from build123d import *

# Parameters (mm, degrees)
SKETCH2_W           = 24
SKETCH2_H           = 24
BOSS_EXTRUDE2_DEPTH = 50
SKETCH4_R           = 1.4
CUT_EXTRUDE1_DEPTH  = 8
CHAMFER1_SIZE       = 2
CHAMFER2_SIZE       = 4


with BuildPart() as part:
    # Sketch2 → Boss-Extrude2 (new body)
    with BuildSketch(Plane.XY):
        with Locations((12, 12)):
            Rectangle(SKETCH2_W, SKETCH2_H)
    extrude(amount=BOSS_EXTRUDE2_DEPTH)

    # Sketch4 → Cut-Extrude1 (cut)
    with BuildSketch(Plane(origin=(0, 0, 0), x_dir=(-1, 0, 0), z_dir=(0, 0, -1))):
        with Locations((-21, 21)):
            Circle(SKETCH4_R)
        with Locations((-21, 3)):
            Circle(SKETCH4_R)
        with Locations((-3, 3)):
            Circle(SKETCH4_R)
        with Locations((-3, 21)):
            Circle(SKETCH4_R)
    extrude(amount=-CUT_EXTRUDE1_DEPTH, mode=Mode.SUBTRACT)

    # Chamfer1
    chamfer1_edges = [part.edges().sort_by_distance(p)[0] for p in [
        (0, 24, 25),
        (24, 24, 25),
        (24, 0, 25),
        (0, 0, 25),
    ]]
    chamfer(chamfer1_edges, length=CHAMFER1_SIZE)

    # Chamfer2
    # the kernel refuses this chamfer: 4 mm, written as the material it takes off along each edge
    with BuildSketch(Plane(origin=(-8.286731952, 0, 50), x_dir=(0, -0.02749587661058639, -0.9996219169112968), z_dir=(1, 0, 0))) as chamfer2_piece_1:
        Polygon((CHAMFER2_SIZE * 0.999621916911, CHAMFER2_SIZE * 0.0274958766106), (-CHAMFER2_SIZE * 0.0274958766106, CHAMFER2_SIZE * 0.999621916911), (0, 0), align=None)
    extrude(amount=40.573463904, mode=Mode.SUBTRACT)
    with BuildSketch(Plane(origin=(24, -8.286731952, 50), x_dir=(-0.9996219169112968, 0, 0.027495876610585623), z_dir=(0, 1, 0)), Plane(origin=(32.286731952, 24, 50), x_dir=(0, -0.9996219169112968, 0.027495876610585623), z_dir=(-1, 0, 0)), Plane(origin=(0, 32.286731952, 50), x_dir=(0.9996219169112968, 0, 0.02749587661058563), z_dir=(0, -1, 0))) as chamfer2_piece_2:
        Polygon((CHAMFER2_SIZE * 0.999621916911, -CHAMFER2_SIZE * 0.0274958766106), (-CHAMFER2_SIZE * 0.0274958766106, -CHAMFER2_SIZE * 0.999621916911), (0, 0), align=None)
    extrude(amount=40.573463904, mode=Mode.SUBTRACT)


solid = part.part
Geometry: final body of the model. Coordinates: model frame, mm. A direction names the side the tool comes from. Give positions to 0.01 mm unless a question says otherwise; leave off trailing zeros. Loops run counter-clockwise (first coordinate to the right, second up) from the corner with the lowest first, then second, coordinate; pieces in that order, holes last. Notation, with made-up numbers: M 16.25,59 L 22.25,59 A24 ccw 22.25,80 Z; hole C -21,39.5 d7. An arc over 180 degrees is marked long. Put each result on its own line as item: value. Start each with the question number.
1) Pull-direction query (Y, two-part tool) for faces 1 (the flat face through (23, 1, 23)), 2 (the cylindrical face through (20.35, 19.76, 3.94)), 3 (the flat face through (12, 24, 23)), 4 (the cylindrical face through (3.303, 19.633, 3.944)); classes: pulls with the +Y half, pulls with the -Y half, needs draft (parallel to the pull), parting line crosses it, or undercut.
2) Cut plane A-A (z = 3.5). Output: boundary loops of the cut face in (x, y).
3) Ray query, line 1 along Y through (x, z) = (21, 4.75); line 2 along Y through (x, z) = (11, 48); line 3 along Z through (x, y) = (22, 16.5). Return the intervals inside material, ascending.
4) Cut plane B-B (y = 21). Output: boundary loops of the cut face in (x, z).
5) Access query for faces 5 (the flat face through (3, 3, 8)), 6 (the flat face through (12, 12, 0)). Directions: +Z, -Z, +X, -X, +Y, -Y. A direction counts if a zero-diameter tool reaches every point of the face in a straight line with its end or side. Return the directions, or none.
6) Contact query for flat-ended pins moving along their axis: pin 1 (1.4 mm diameter, centred on x = 3, y = 21, fed in from -Z); pin 2 (2 mm diameter, centred on x = 21, y = 3, fed in from +Z). Output: stop coordinate, or through.
Verdict:
1. face 1: pulls with the -Y half
1. face 2: undercut
1. face 3: pulls with the +Y half
1. face 4: undercut
2. outline: M 0,2 L 2,0 L 22,0 L 24,2 L 24,22 L 22,24 L 2,24 L 0,22 Z; hole C 3,3 d2.8; hole C 3,21 d2.8; hole C 21,3 d2.8; hole C 21,21 d2.8
3. line 1: 0 to 1.6, 4.4 to 19.6, 22.4 to 24
3. line 2: 2 to 22
3. line 3: 0 to 48
4. outline: M 0,0 L 1.6,0 L 1.6,8 L 4.4,8 L 4.4,0 L 19.6,0 L 19.6,8 L 22.4,8 L 22.4,0 L 24,0 L 24,46 L 21,49 L 3,49 L 0,46 Z
5. face 5: -Z
5. face 6: -Z, +X, -X, +Y, -Y
6. pin 1: z = 8
6. pin 2: z = 49.71
